Autodesk Inventor part; units mm, degrees
ref_plane "YZ Plane" through (0, 0, 0) normal (1, 0, 0) x (0, 1, 0)
ref_plane "XZ Plane" through (0, 0, 0) normal (0, 1, 0) x (-1, 0, 0)
ref_plane "XY Plane" through (0, 0, 0) normal (0, 0, 1) x (1, 0, 0)
sketch "Sketch1" plane through (0, 0, 0) normal (0, 0, 1) x (1, 0, 0)
  line L0 (-15.5, 15.5) -> (15.5, 15.5) construction
  line L1 (15.5, 15.5) -> (15.5, -15.5) construction
  line L2 (15.5, -15.5) -> (-15.5, -15.5) construction
  line L3 (-15.5, -15.5) -> (-15.5, 15.5) construction
  line L4 (-15.5, 15.5) -> (15.5, -15.5) construction
  line L5 (15.5, 15.5) -> (-15.5, -15.5) construction
  circle A0 centre (0, 0) radius 11.5
  circle A1 centre (15.5, 15.5) radius 1.75
  circle A2 centre (15.5, -15.5) radius 1.75
  circle A3 centre (-15.5, -15.5) radius 1.75
  circle A4 centre (-15.5, 15.5) radius 1.75
  line L6 (-21.5, -21.5) -> (21.5, -21.5)
  line L7 (21.5, -21.5) -> (21.5, 21.5)
  line L8 (21.5, 21.5) -> (-21.5, 21.5)
  line L9 (-21.5, 21.5) -> (-21.5, -21.5)
  line L10 (-21.5, -21.5) -> (21.5, 21.5) construction
  line L11 (21.5, -21.5) -> (-21.5, 21.5) construction
  dimension "d0" = 23
  dimension "d1" = 3.5
  dimension "d2" = 31
  dimension "d3" = 31
  dimension "d4" = 43
extrude "Extrusion1" add sketch "Sketch1" against normal mid plane 4
sketch "Sketch2" plane through (-21.5, -21.5, -2) normal (-1, 0, 0) x (0, 0, 1)
  line L0 (0, 43) -> (4, 43)
  line L1 (0, 0) -> (0, 43)
  line L2 (0, 0) -> (4, 0)
  line L3 (4, 43) -> (4, 0)
  line L4 (0, 43) -> (4, 43)
  line L5 (0, 43) -> (-28, 4)
  line L6 (-28, 4) -> (-28, 0)
  line L7 (0, 43) -> (0, 0)
  line L8 (-28, 0) -> (0, 0)
  point P0 (2, 21.5)
  dimension "d7" = 28
  dimension "d8" = 4
extrude "Extrusion2" add sketch "Sketch2" along normal blind 3
sketch "Sketch3" plane through (21.5, -21.5, -2) normal (1, 0, 0) x (0, 0, -1)
  line L0 (-4, 0) -> (0, 0)
  line L1 (0, 43) -> (0, 0)
  line L2 (0, 43) -> (-4, 43)
  line L3 (-4, 0) -> (-4, 43)
  line L4 (-4, 0) -> (-4, 43)
  line L5 (-4, 43) -> (-29, 4)
  line L6 (-29, 4) -> (-29, 0)
  line L7 (-29, 0) -> (-4, 0)
  point P0 (-2, 21.5)
  dimension "d11" = 4
  dimension "d12" = 25
extrude "Extrusion3" add sketch "Sketch3" along normal blind 3
sketch "Sketch4" plane through (-21.5, -21.5, -30) normal (0, -1, 0) x (1, 0, 0)
  arc A0 (39.5, 57) -> (39.5, 50) centre (39.5, 53.5) ccw
  line L0 (43, 32) -> (43, 57)
  line L1 (43, 57) -> (39.5, 57)
  line L2 (39.5, 50) -> (43, 50)
  line L3 (39.5, 50) -> (39.5, 57) construction
  circle A1 centre (39.5, 53.5) radius 1.75
  arc A2 (-6.5, 32) -> (-6.5, 25) centre (-6.5, 28.5) ccw
  line L4 (-3, 32) -> (-6.5, 32)
  line L5 (-6.5, 25) -> (-3, 25)
  line L6 (-6.5, 25) -> (-6.5, 32) construction
  circle A3 centre (-6.5, 28.5) radius 1.75
  arc A4 (-6.5, 7) -> (-6.5, 0) centre (-6.5, 3.5) ccw
  line L7 (-3, 7) -> (-6.5, 7)
  line L8 (-6.5, 0) -> (-3, 0)
  line L9 (-6.5, 0) -> (-6.5, 7) construction
  circle A5 centre (-6.5, 3.5) radius 1.75
  line L10 (-3, 0) -> (-3, 32)
  arc A6 (16.5, 35.5) -> (9.5, 35.5) centre (13, 35.5) ccw
  line L11 (16.5, 32) -> (16.5, 35.5)
  line L12 (9.5, 35.5) -> (9.5, 32)
  line L13 (9.5, 35.5) -> (16.5, 35.5) construction
  circle A7 centre (13, 35.5) radius 1.75
  line L14 (43, 32) -> (-3, 32)
  line L15 (0, 28) -> (46, 28)
  line L16 (46, 32) -> (46, 57)
  point P0 (21.5, 30)
  dimension "d15" = 3.5
  dimension "d16" = 3.5
  dimension "d19" = 3.5
  dimension "d20" = 3.5
  dimension "d21" = 3.5
  dimension "d22" = 3.5
  dimension "d23" = 3.5
  dimension "d24" = 3.5
  dimension "d25" = 16
  dimension "d27" = 25.5
  dimension "d28" = 6.5
  dimension "d31" = 26.5
  dimension "d32" = 19.5
  dimension "d33" = 18
  dimension "d34" = 7
  dimension "d35" = 25
extrude "Extrusion4" add sketch "Sketch4" against normal blind 4
fillet "Fillet1" radius 2 5 edges at (-24.5, -19.5, -23) (-12, -19.5, 2) (-24.5, -19.5, -5) (-5, -19.5, 2) (21.5, -19.5, 20)
fillet "Fillet2" radius 5 1 edges at (-21.5, -19.5, -30)
properties part number "PitchMotorBracket"
The listing builds one solid part. Answer for the finished solid, in the listing's coordinates (mm). A direction names the side the tool comes from. Round coordinates to 2 decimals unless told otherwise and drop trailing zeros. Write each loop counter-clockwise with the first axis right and the second up, starting at its lowest first coordinate (ties: lowest second). Pieces come first, ordered by that corner, then holes. Notation, with made-up numbers: (54.25, 72.25) -> (85.25, 72.25) arc R28 cw to (85.25, 109.25) -> close; hole circle Ø11 at (-16.5, 89.25). An arc over 180 degrees is marked (long way). Use CSV: the item, a comma, the result in double quotes. Start each with the question number.
(1) Each of these flat-tipped pins is pushed along its axis until it touches: pin 1 (3.5 mm diameter, centred on x = -8.5, z = 4.5, fed in from +Y); pin 2 (16 mm diameter, centred on y = -4.5, z = -15, fed in from -X); pin 3 (4 mm diameter, centred on x = -15.5, y = 15.5, fed in from -Z). Where does it stop, or does it pass through?
(2) Section C-C on x = 4.5 is taken. Give the vertices of the cut face in (y, z), then the cut area to 3 significant figures.
(3) Section D-D on y = 15.5 is taken. Give the vertices of the cut face in (x, z).
(4) Section A-A on z = 23.5 is taken. Give the vertices of the cut face in (x, y), then the cut area to 3 significant figures.
(5) Which of the six approach directions +Z, -Z, +X, -X, +Y, -Y give full straight-line access (tool end or side, diameter ignored) to faces 5 (the face through (-25.1, -19.47, -5.57)), 6 (the face through (-21.5, -4, -11)), 7 (the face through (-7, -17.5, 4)), 8 (the face through (-4.4, -19.47, 2.57)), 9 (the face through (-26, -17.5, -2))?
(6) Section B-B on y = -14.5 is taken. Give the vertices of the cut face in (x, z), then the cut area to 3 significant figures.
(7) The mould has two halves that part along Z. Classify faces 1 (the face through (22.979, 2.273, 14.325)), 2 (the face through (11, -4, -2)), 3 (the face through (-7.69, -19.53, 3.95)), 4 (the face through (-1.5, -11.4, 0)): released by +Z, released by -Z, zero draft, split by the parting line, or undercut.
(8) Consider L1, parallel to Z at x = -28, y = -19.6; L2, parallel to X at y = -20, z = 5; L3, parallel to X at y = 15, z = 0. Determine where each line is inside the solid, lowest interval first. Write a range as from..to.
A:
1,pin 1,"stops at y = -17.5"
1,pin 2,"stops at x = -24.5"
1,pin 3,"stops at z = -2"
2,outline,"(-21.5, -2) -> (-10.58, -2) -> (-10.58, 2) -> (-21.5, 2) -> close; (10.58, -2) -> (21.5, -2) -> (21.5, 2) -> (10.58, 2) -> close"
2,area,"87.3 mm²"
3,outline,"(-24.5, -6.31) -> (-21.5, -6.31) -> (-21.5, -2) -> (-17.25, -2) -> (-17.25, 2) -> (-24.5, 2) -> close; (-13.75, -2) -> (13.75, -2) -> (13.75, 2) -> (-13.75, 2) -> close; (17.25, -2) -> (24.5, -2) -> (24.5, 5.85) -> (21.5, 5.85) -> (21.5, 2) -> (17.25, 2) -> close"
4,outline,"(14.5, -21.5) -> (16.25, -21.5) -> (16.25, -17.5) -> (14.5, -17.5) -> close; (19.75, -21.5) -> (24.5, -21.5) -> (24.5, -12.04) -> (21.5, -12.04) -> (21.5, -17.5) -> (19.75, -17.5) -> close"
4,area,"42.4 mm²"
5,face 5,"-X, +Y, -Y"
5,face 6,"-Z, +X, +Y, -Y"
5,face 7,"+Z, -X, +Y"
5,face 8,"+Z, +Y, -Y"
5,face 9,"+Z, -Z, -X, +Y"
6,outline,"(-24.5, -27.85) -> (-22.39, -27.85) arc R5 ccw to (-21.5, -25) -> (-21.5, -2) -> (-16.94, -2) -> (-16.94, 2) -> (-24.5, 2) -> close; (-14.06, -2) -> (14.06, -2) -> (14.06, 2) -> (-14.06, 2) -> close; (16.94, -2) -> (24.5, -2) -> (24.5, 25.08) -> (21.5, 25.08) -> (21.5, 2) -> (16.94, 2) -> close"
6,area,"319 mm²"
7,face 1,"released by +Z"
7,face 2,"released by -Z"
7,face 3,"undercut"
7,face 4,"zero draft"
8,L1,"z = -30..-28.25, -24.75..-23, -5..-3.25, 0.25..2"
8,L2,"x = -12..-10.18, -6.82..-5, 21.5..24.5"
8,L3,"x = -24.5..-17.18, -13.82..13.82, 17.18..24.5"
